Input: part model. Units: mm. Frame: model coordinates. Face numbers are marked on the shaded views. A direction names the side the tool comes from. Round coordinates to 2 decimals unless told otherwise and drop trailing zeros. Loops run counter-clockwise (first coordinate to the right, second up) from the corner with the lowest first, then second, coordinate; pieces in that order, holes last.
(1) Cut plane B-B, the plane y = -19.05. Output: boundary loops of the cut face in (x, z).
(2) Cut plane A-A, the plane x = 50.8. Output: boundary loops of the cut face in (y, z), and give its area (3 significant figures).
(3) Cut plane C-C, the plane z = 228.6. Output: boundary loops of the cut face in (x, y).
(4) Line query: line 1 (X direction, y = -19, z = 10); line 2 (X direction, y = -4, z = 228); line 3 (Z direction, x = 114.3, y = -4.75). Output: solid intervals per line, ascending.
(5) Cut plane D-D, the plane x = 12. Output: boundary loops of the cut face in (y, z).
(6) Access query for the marked faces 1 and 2. Directions: +Z, -Z, +X, -X, +Y, -Y. A direction counts if a zero-diameter tool reaches every point of the face in a straight line with its end or side. Return the directions, or none.
(7) First-contact query: pin 1 Ø5 at (x, z) = (34.5, 189) entering from -Y; pin 2 Ø12 at (x, y) = (34.925, -19.05) entering from -Z; pin 3 Ø7.5 at (x, y) = (107, -23.5) entering from +Z. Flat tips, straight axial feed; report the tip coordinate or a pass-through.
from build123d import *

# Parameters (mm, degrees)
F1_DEPTH = 6.35
F3_D     = 13.49248
F4_W     = 165.1
F4_H     = 12.7
F5_DEPTH = 25.4
F6_R     = 5.08
F8_D     = 13.49248


with BuildPart() as f1:
    # F0 (on Front) → F1 (new body)
    with BuildSketch(Plane.XZ):
        with BuildLine():
            Line((0, 241.3), (0, 0))
            Line((0, 0), (165.1, 0))
            Line((165.1, 0), (165.1, 241.3))
            ThreePointArc((165.1, 241.3), (157.6605122421, 259.2605122421), (139.7, 266.7))
            Line((139.7, 266.7), (25.4, 266.7))
            ThreePointArc((25.4, 266.7), (7.4394877579, 259.2605122421), (0, 241.3))
        make_face()
    extrude(amount=F1_DEPTH)

    # F3 (through all)
    with Locations(Plane.XZ.offset(6.35)):
        with Locations((50.8, 228.6), (114.3, 228.6)):
            Hole(F3_D / 2)

    # F4 (on face) → F5 (join)
    with BuildSketch(Plane.XZ.offset(6.35)):
        with Locations((82.55, 6.35)):
            Rectangle(F4_W, F4_H)
    extrude(amount=F5_DEPTH)

    # F6
    f6_edges = [f1.edges().sort_by_distance(p)[0] for p in [
        (165.1, -31.75, 6.35),
        (0, -31.75, 6.35),
    ]]
    fillet(f6_edges, radius=F6_R)

    # F8 (through all)
    with Locations(Plane.XY.offset(12.7)):
        with Locations((34.925, -19.05), (130.175, -19.05)):
            Hole(F8_D / 2)


solid = f1.part
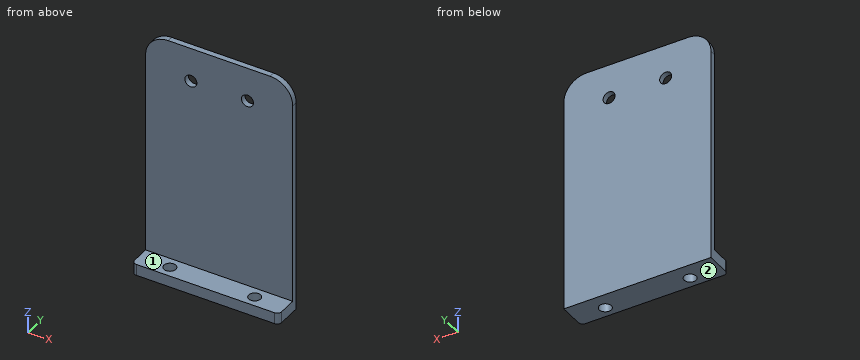
Reported:
1. outline: (0, 0) - (28.18, 0) - (28.18, 12.7) - (0, 12.7) - close; (41.67, 0) - (123.43, 0) - (123.43, 12.7) - (41.67, 12.7) - close; (136.92, 0) - (165.1, 0) - (165.1, 12.7) - (136.92, 12.7) - close
2. outline: (-31.75, 0) - (0, 0) - (0, 221.85) - (-6.35, 221.85) - (-6.35, 12.7) - (-31.75, 12.7) - close; (-6.35, 235.35) - (0, 235.35) - (0, 266.7) - (-6.35, 266.7) - close
2. area: 1,930 mm2
3. outline: (0, -6.35) - (44.05, -6.35) - (44.05, 0) - (0, 0) - close; (57.55, -6.35) - (107.55, -6.35) - (107.55, 0) - (57.55, 0) - close; (121.05, -6.35) - (165.1, -6.35) - (165.1, 0) - (121.05, 0) - close
4. line 1: x = 0 to 28.18, 41.67 to 123.43, 136.92 to 165.1
4. line 2: x = 0 to 44.08, 57.52 to 107.58, 121.02 to 165.1
4. line 3: z = 0 to 221.85, 235.35 to 266.7
5. outline: (-31.75, 0) - (0, 0) - (0, 262.88) - (-6.35, 262.88) - (-6.35, 12.7) - (-31.75, 12.7) - close
6. face 1: +Z, +X, -X, -Y
6. face 2: -Z, +X, -X, +Y, -Y
7. pin 1: stops at y = -6.35
7. pin 2: passes through
7. pin 3: stops at z = 12.7
